The listing builds one solid part. Answer for the finished solid, in the listing's coordinates (mm). Face numbers are marked on the shaded views. A direction names the side the tool comes from. Give positions to 0.01 mm unless a question says otherwise; leave off trailing zeros. Write each loop counter-clockwise with the first axis right and the second up, starting at its lowest first coordinate (ties: lowest second). Pieces come first, ordered by that corner, then holes. Notation, with made-up numbers: (39, 11) - (50, 11) arc R15 ccw to (50, 23) - close; hole circle Ø5 at (52.5, 72.5). An arc over 180 degrees is marked (long way). Return JSON: item names as keys, results as strings.
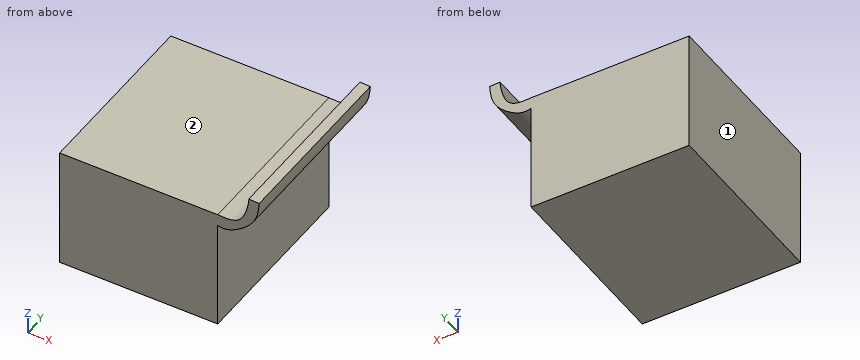
from build123d import *

# Parameters (mm, degrees)
F1_DEPTH = 150


with BuildPart() as f1:
    # F0 (on Front) → F1 (new body)
    with BuildSketch(Plane.XZ):
        with BuildLine():
            Line((66.5512742102, 53.22832472), (-63.4487257898, 53.22832472))
            Line((-63.4487257898, 53.22832472), (-63.4487257898, -46.77167528))
            Line((-63.4487257898, -46.77167528), (66.5512742102, -46.77167528))
            Line((66.5512742102, -46.77167528), (66.5512742102, 43.4356927872))
            add(Edge.make_bspline(
                [(66.5512742102, 43.4356927872), (69.0458437789, 42.8412241475), (75.8185758553, 41.2272475823), (98.8077186481, 57.2419967752), (100.0567297058, 71.5116963556), (100.6503552198, 78.2937481999)],
                knots=[0, 0, 0, 0, 0.2342815252, 0.6360720585, 1, 1, 1, 1], degree=3))
            Line((100.6503552198, 78.2937481999), (92.0727178454, 78.6587521434))
            add(Edge.make_bspline(
                [(66.5512742102, 53.22832472), (74.1004513767, 52.7601957711), (89.292724355, 51.8181139225), (92.4721770478, 78.2514275942), (92.0727178454, 78.6587521434)],
                knots=[0, 0, 0, 0, 0.4706037901, 0.9470623203, 0.9470623203, 0.9470623203, 0.9470623203], degree=3))
        make_face()
    extrude(amount=F1_DEPTH)


solid = f1.part
Item 1: Flat-ended cylindrical pins translate along their axes: P1, Ø1.5, axis at y = -19.5, z = 11.5, coming from the +X side; P2, Ø1, axis at x = 24.5, y = -54, coming from the +Z side. Find the tip coordinate at first contact, or state that the pin passes through.
Answer below:
{"P1": "stops at x = 66.55", "P2": "stops at z = 53.23"}
Item 2: A cutting plane is placed at B-B on z = 34. Determine the outline of the cut face in (x, y).
Answer below:
{"outline": "(-63.45, -150) - (66.55, -150) - (66.55, 0) - (-63.45, 0) - close"}
Item 3: A cutting plane is placed at A-A on x = 25. Determine the outline of the cut face in (y, z).
Answer below:
{"outline": "(-150, -46.77) - (0, -46.77) - (0, 53.23) - (-150, 53.23) - close"}
Item 4: For the marked faces 1 and 2, determine the directions among +Z, -Z, +X, -X, +Y, -Y from which every point of the face is accessible in a straight line to the end or side of a thin tool.
Answer below:
{"face 1": "+Z, -Z, -X, +Y, -Y", "face 2": "+Z, -X, +Y, -Y"}
Item 5: Consider L1, parallel to Z at x = -6, y = -122; L2, parallel to X at y = -47, z = -16; L3, parallel to X at y = -8.5, z = 49. Determine where each line is inside the solid, lowest interval first.
Answer below:
{"L1": "z = -46.77 to 53.23", "L2": "x = -63.45 to 66.55", "L3": "x = -63.45 to 85.85"}
